The figure shows three views and two pictorial views of one solid part (mm, origin at its lowest corner). Answer the questions. Coordinates: 2 decimals unless noted, no trailing zeros. Order: outer loops, then holes, each group sorted by start corner. A loop starts at its lowest first (then second) coordinate and runs counter-clockwise, first axis right, second up. Notation, with made-up numbers: M 21.25,-12.75 L 74.25,-12.75 A23 ccw 74.25,22.25 Z; hole C -14.75,-20.5 d11. An arc over 180 degrees is marked long. Use a Markdown table: item, result.
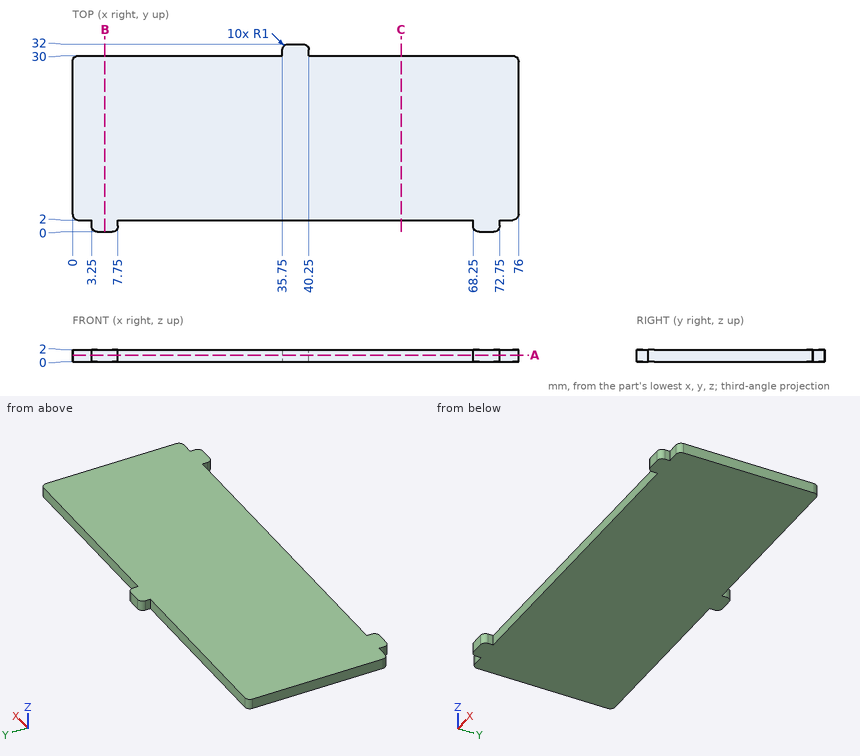
1. Find the intervals of material crossed by probe 1 along Y at (x, z) = (65, 0.35); probe 2 along X at (y, z) = (2.5, 1.55); probe 3 along Y at (x, z) = (40, 0.25), in increasing order.
Answers below:
| item | result |
|---|---|
| probe 1 | 2 to 30 |
| probe 2 | 0.13 to 75.87 |
| probe 3 | 2 to 31.66 |
2. Section C-C on x = 56 is taken. Determine the outline of the cut face in (y, z).
Answers below:
| item | result |
|---|---|
| outline | M 2,0 L 30,0 L 30,2 L 2,2 Z |
3. Section B-B on x = 5.5 is taken. Determine the outline of the cut face in (y, z), then the cut area to 3 significant figures.
Answers below:
| item | result |
|---|---|
| outline | M 0,0 L 30,0 L 30,2 L 0,2 Z |
| area | 60.0 mm² |
4. Section A-A on z = 1.1 is taken. Determine the outline of the cut face in (x, y).
Answers below:
| item | result |
|---|---|
| outline | M 0,3 A1 ccw 1,2 L 3.25,2 L 3.25,1 A1 ccw 4.25,0 L 6.75,0 A1 ccw 7.75,1 L 7.75,2 L 68.25,2 L 68.25,1 A1 ccw 69.25,0 L 71.75,0 A1 ccw 72.75,1 L 72.75,2 L 75,2 A1 ccw 76,3 L 76,29 A1 ccw 75,30 L 40.25,30 L 40.25,31 A1 ccw 39.25,32 L 36.75,32 A1 ccw 35.75,31 L 35.75,30 L 1,30 A1 ccw 0,29 Z |
5. Flat-ended cylindrical pins translate along their axes: P1, Ø1, axis at x = 41.5, z = 0.5, coming from the +Y side; P2, Ø0.6, axis at x = 44, z = 1, coming from the -Y side; P3, Ø0.8, axis at y = 30.5, z = 1.5, coming from the +X side. Find the tip coordinate at first contact, or state that the pin passes through.
Answers below:
| item | result |
|---|---|
| P1 | y = 30 |
| P2 | y = 2 |
| P3 | x = 40.25 |
